Build history of the part. All positions in model axes, mm. Face numbers are marked on the shaded views. Round coordinates to 2 decimals unless told otherwise and drop trailing zeros. Write each loop counter-clockwise with the first axis right and the second up, starting at its lowest first coordinate (ties: lowest second). Pieces come first, ordered by that corner, then holes.
1) Wall check: probe 1 along X at (y, z) = (-11.5, 4.5); probe 2 along Y at (x, z) = (-6, 7.75); probe 3 along Y at (x, z) = (-22, 9). Give the ranges that are in metal, low to high.
2) Flat gauge pin, fed straight in: pin 1 (5 mm diameter, centred on x = 64.5, z = 6.5, fed in from +Y). Where does the tip first touch, or does it go through?
3) Saw through at D-D (x = 66). Write the cut outline in (y, z) (3 decimals), plus the area to 3 significant figures.
4) Pull direction X, two halves, no side cores. Call the marked faces 1, 2 and 3: +X half, -X half, draft (parallel to the pull), parting line (faces both ways), or undercut.
5) Saw through at A-A (x = -22). Write the cut outline in (y, z), plus the area to 3 significant figures.
6) Saw through at B-B (y = -15). Write the cut outline in (x, z) (3 decimals).
7) Saw through at C-C (z = 6). State how many separate pieces and enclosed holes the cut face has, plus the area to 3 significant figures.
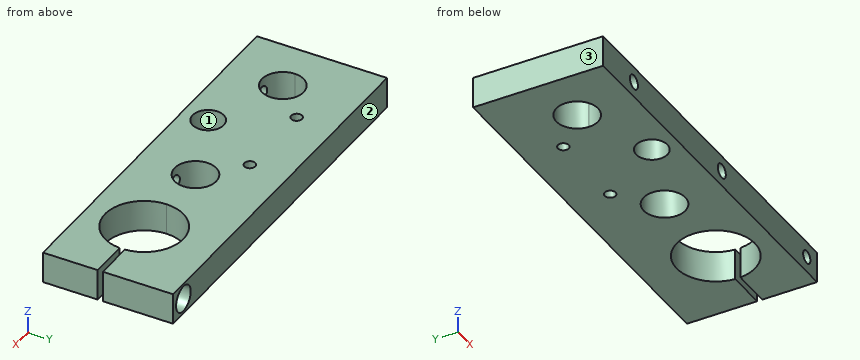
from build123d import *

# Parameters (mm, degrees)
F0_R           = 2.1
F0_R_2         = 6
F1_DEPTH       = 12
F3_D           = 4.91
F3_DEPTH       = 27
F5_D           = 6
F5_DEPTH       = 27
F5_CBORE_D     = 10
F5_CBORE_DEPTH = 15
F7_D           = 5.48
F7_DEPTH       = 20


with BuildPart() as f1:
    # F0 (on Top) → F1 (new body)
    with BuildSketch(Plane.XY):
        with BuildLine():
            Line((-73, 25), (-73, -3))
            Line((-73, -3), (-59.997182, -3))
            ThreePointArc((-59.997182, -3), (-52, 4.787677), (-44.002818, -3))
            Line((-44.002818, -3), (0, -3))
            ThreePointArc((0, -3), (8, 5), (16, -3))
            Line((16, -3), (27.95, -3))
            ThreePointArc((27.95, -3), (42.499724, 12.041683), (58.016741, -2))
            Line((58.016741, -2), (73, -2))
            Line((73, -2), (73, 25))
            Line((73, 25), (-73, 25))
        make_face()
        with Locations((-38, 10)):
            Circle(F0_R, mode=Mode.SUBTRACT)
        with Locations((-6, 10)):
            Circle(F0_R, mode=Mode.SUBTRACT)
        with BuildLine():
            Line((-73, -25), (73, -25))
            Line((73, -25), (73, -4))
            Line((73, -4), (58.016741, -4))
            ThreePointArc((58.016741, -4), (42.499724, -18.041683), (27.95, -3))
            Line((27.95, -3), (16, -3))
            ThreePointArc((16, -3), (8, -11), (0, -3))
            Line((0, -3), (-44.002818, -3))
            ThreePointArc((-44.002818, -3), (-44.000705, -3.106152), (-44, -3.212323))
            ThreePointArc((-44, -3.212323), (-52.106171, -11.211619), (-59.997182, -3))
            Line((-59.997182, -3), (-73, -3))
            Line((-73, -3), (-73, -25))
        make_face()
        with Locations((-22, -15)):
            Circle(F0_R_2, mode=Mode.SUBTRACT)
    extrude(amount=F1_DEPTH)

    # F3
    with Locations(Plane.XZ.offset(25)):
        with Locations((66, 6)):
            Hole(F3_D / 2, depth=F3_DEPTH)

    # F5
    with Locations(Plane(origin=(0, 25, 0), x_dir=(-1, 0, 0), z_dir=(0, 1, 0))):
        with Locations((-66, 6)):
            CounterBoreHole(F5_D / 2, F5_CBORE_D / 2, F5_CBORE_DEPTH, depth=F5_DEPTH)

    # F7
    with Locations(Plane.XZ.offset(25)):
        with Locations((-52, 6), (8, 6)):
            Hole(F7_D / 2, depth=F7_DEPTH)


solid = f1.part
Evaluation:
1. probe 1: x = -73 to -54.29, -49.71 to -26.87, -17.13 to 5.71, 10.29 to 30.58, 55.42 to 64.06, 67.94 to 73
1. probe 2: y = -25 to 7.9, 12.1 to 25
1. probe 3: y = -25 to -21, -9 to 25
2. pin 1: stops at y = 10
3. outline: (-25, 0) - (-4, 0) - (-4, 3.545) - (-25, 3.545) - close; (-25, 8.455) - (-4, 8.455) - (-4, 12) - (-25, 12) - close; (-2, 0) - (25, 0) - (25, 1) - (10, 1) - (10, 3) - (-2, 3) - close; (-2, 9) - (10, 9) - (10, 11) - (25, 11) - (25, 12) - (-2, 12) - close
3. area: 251 mm2
4. face 1: undercut
4. face 2: draft
4. face 3: -X half
5. outline: (-25, 0) - (-21, 0) - (-21, 12) - (-25, 12) - close; (-9, 0) - (25, 0) - (25, 12) - (-9, 12) - close
5. area: 456 mm2
6. outline: (-73, 0) - (-28, 0) - (-28, 12) - (-73, 12) - close; (-16, 0) - (33.917, 0) - (33.917, 12) - (-16, 12) - close; (52.083, 0) - (73, 0) - (73, 12) - (52.083, 12) - close; hole circle Ø5.48 at (-52, 6); hole circle Ø5.48 at (8, 6); hole circle Ø4.91 at (66, 6)
7. separate pieces: 3
7. enclosed holes: 3
7. area: 5,540 mm2
